Here's how the part is built. I have some questions about the finished solid (model axes, mm). A direction names the side the tool comes from. Give positions to 0.01 mm unless a question says otherwise; leave off trailing zeros. Order: outer loops, then holes, each group sorted by start corner. A loop starts at its lowest first (then second) coordinate and runs counter-clockwise, first axis right, second up. Notation, with made-up numbers: (-1.5, -13.75) -> (6.5, -13.75) arc R22 cw to (6.5, 12.25) -> close; hole circle Ø3 at (67, -23.75). An arc over 180 degrees is marked (long way). Write each question's results on one line, items separated by ' | '. Start each with the question number.
Q1. Imagine slicing it at D-D, the plane y = 19. Please give me the cut outline in (x, z), then the cut area to 3 significant figures.
Q2. I need wall thicknesses on line 1 along Y through (x, z) = (4, 0.65); line 2 along X through (y, z) = (12.25, 0.8); line 3 along X through (y, z) = (3.5, 2.6). Which ranges of each line are inside material? Lowest first, please. Write a range as [from, to].
Q3. For faces 1 (the face through (11.998, 13, 2)), 2 (the face through (17.984, 12.226, 1.521)), which set-ups out of +Z, -Z, +X, -X, +Y, -Y let a thin tool reach every point of the face, with its end or its side?
Q4. I'm going to push flat-ended pins straight in: pin 1 (0.6 mm diameter, centred on x = 10.5, z = 2, fed in from -Y); pin 2 (0.6 mm diameter, centred on x = 11, z = 1, fed in from +Y); pin 3 (0.9 mm diameter, centred on y = 7.5, z = 2, fed in from -X). Where does each tip first touch, or does it pass through?
Q5. Imagine slicing it at C-C, the plane z = 2.3. Please give me the cut outline in (x, y).
Q6. Imagine slicing it at A-A, the plane x = 2. Please give me the cut outline in (y, z), then the cut area to 3 significant figures.
Q7. Imagine slicing it at B-B, the plane y = 8.5. Please give me the cut outline in (x, z), then the cut area to 3 significant figures.
Q8. Thinking about a two-plate mould opening in X: for faces 3 (the face through (-21, 12.8, 1.5)), 4 (the face through (11, 10.001, 2)), 5 (the face through (-2, 18.6, 2)), 6 (the face through (-6, 4, 0)), which applies, pulls with the +X half, pulls with the -X half, needs draft (parallel to the pull), parting line crosses it, or undercut?
```python
from build123d import *

# Parameters (mm, degrees)
SKETCH_1_R      = 1.3
EXTRUDE_1_DEPTH = 3


with BuildPart() as part:
    # 草图1 → 凸台-拉伸1 (new body)
    with BuildSketch(Plane.XY.offset(3)):
        with BuildLine():
            Line((-8.503322156, 0.0005), (5.486588529, 0.0005))
            ThreePointArc((5.486588529, 0.0005), (17.986588529, 12.5005), (5.486588529, 25.0005))
            Line((5.486588529, 25.0005), (-8.503322156, 25.0005))
            ThreePointArc((-8.503322156, 25.0005), (-21.003322156, 12.5005), (-8.503322156, 0.0005))
        make_face()
        with Locations(Location((-1.487905971, 2.9995, 0), (0, 0, 180))):
            Circle(SKETCH_1_R, mode=Mode.SUBTRACT)
        with Locations(Location((-1.487905971, 22.0005, 0), (0, 0, 180))):
            Circle(SKETCH_1_R, mode=Mode.SUBTRACT)
        Polygon((11.997794717, 15), (11.997794717, 10.001), (9.996894717, 10.001), (9.996894717, 6.4), (-13.002605283, 6.4), (-13.002605283, 18.6), (9.996894717, 18.6), (9.996894717, 15), align=None, mode=Mode.SUBTRACT)
    extrude(amount=-EXTRUDE_1_DEPTH)


solid = part.part
```
Geometry check:
1) outline: (-19.18, 0) -> (16.16, 0) -> (16.16, 3) -> (-19.18, 3) -> close | area: 106 mm²
2) line 1: [0, 6.4], [18.6, 25] | line 2: [-21, -13], [12, 17.98] | line 3: [-17.18, -2.69], [-0.29, 14.16]
3) face 1: +Z, -Z | face 2: +Z, -Z, +X
4) pin 1: y = 0.92 | pin 2: y = 23.86 | pin 3: x = -20.15
5) outline: (-8.5, 0) -> (5.49, 0) arc R12.5 ccw to (5.49, 25) -> (-8.5, 25) arc R12.5 ccw to start; hole (-13, 6.4) -> (10, 6.4) -> (10, 10) -> (12, 10) -> (12, 15) -> (10, 15) -> (10, 18.6) -> (-13, 18.6) -> close; hole circle Ø2.6 at (-1.49, 3); hole circle Ø2.6 at (-1.49, 22)
6) outline: (0, 0) -> (6.4, 0) -> (6.4, 3) -> (0, 3) -> close; (18.6, 0) -> (25, 0) -> (25, 3) -> (18.6, 3) -> close | area: 38.4 mm²
7) outline: (-20.35, 0) -> (-13, 0) -> (-13, 3) -> (-20.35, 3) -> close; (10, 0) -> (17.33, 0) -> (17.33, 3) -> (10, 3) -> close | area: 44.0 mm²
8) face 3: pulls with the -X half | face 4: undercut | face 5: undercut | face 6: needs draft
